Geometry check sheet. Reference: the model listing, model coordinates, mm. Round coordinates to 2 decimals unless told otherwise and drop trailing zeros. Order: outer loops, then holes, each group sorted by start corner. A loop starts at its lowest first (then second) coordinate and runs counter-clockwise, first axis right, second up. Notation, with made-up numbers: (17.25, -39.75) - (58.25, -39.75) arc R22 ccw to (58.25, -3.75) - close; hole circle Ø6 at (21, 15.25). An arc over 180 degrees is marked (long way). Write each question's results on one line, items separated by ' | '.
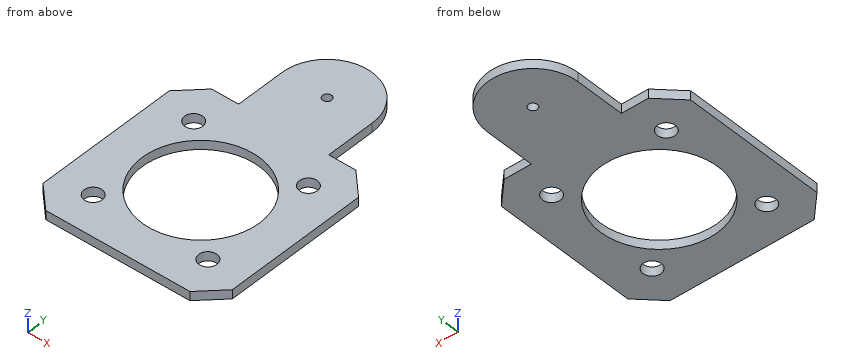
```python
from build123d import *

# Parameters (mm, degrees)
CROQUIS1_R              = 2
CROQUIS1_R_2            = 13
CROQUIS1_R_3            = 1
SALIENTE_EXTRUIR1_DEPTH = 2


with BuildPart() as part:
    # Croquis1 → Saliente-Extruir1 (new body)
    with BuildSketch(Plane.XY):
        with BuildLine():
            Line((10, 21), (16, 21))
            Line((16, 21), (21, 16))
            Line((21, 16), (21, -16))
            Line((21, -16), (16, -21))
            Line((16, -21), (-16, -21))
            Line((-16, -21), (-21, -16))
            Line((-21, -16), (-21, 16))
            Line((-21, 16), (-16, 21))
            Line((-16, 21), (-10, 21))
            Line((-10, 21), (-10, 32))
            ThreePointArc((-10, 32), (0, 42), (10, 32))
            Line((10, 32), (10, 21))
        make_face()
        with Locations((12.727922061, 12.727922061)):
            Circle(CROQUIS1_R, mode=Mode.SUBTRACT)
        with Locations((12.727922061, -12.727922061)):
            Circle(CROQUIS1_R, mode=Mode.SUBTRACT)
        with Locations((-12.727922061, -12.727922061)):
            Circle(CROQUIS1_R, mode=Mode.SUBTRACT)
        with Locations((-12.727922061, 12.727922061)):
            Circle(CROQUIS1_R, mode=Mode.SUBTRACT)
        Circle(CROQUIS1_R_2, mode=Mode.SUBTRACT)
        with Locations((0, 32)):
            Circle(CROQUIS1_R_3, mode=Mode.SUBTRACT)
    extrude(amount=SALIENTE_EXTRUIR1_DEPTH)


solid = part.part
```
(1) Depth check by flat-ended pin: pin 1 Ø2.5 at (x, y) = (12.73, 12.73) entering from +Z. Enter the tip coordinate at first touch or a pass-through.
Answers follow:
pin 1: through
(2) Material ranges on line 1 (Y direction, x = 0, z = 0.4); line 2 (X direction, y = -11.5, z = 1.95); line 3 (Y direction, x = -14, z = 0.3), recorded low to high.
Answers follow:
line 1: -21 to -13, 13 to 31, 33 to 42 | line 2: -21 to -14.31, -11.15 to -6.06, 6.06 to 11.15, 14.31 to 21 | line 3: -21 to -14.27, -11.18 to 11.18, 14.27 to 21
(3) Section check D-D (y = -9.5). Record the cut outline in (x, z).
Answers follow:
outline: (-21, 0) - (-8.87, 0) - (-8.87, 2) - (-21, 2) - close; (8.87, 0) - (21, 0) - (21, 2) - (8.87, 2) - close
(4) Section check A-A (x = 0). Record the cut outline in (y, z), then the cut area to 3 significant figures.
Answers follow:
outline: (-21, 0) - (-13, 0) - (-13, 2) - (-21, 2) - close; (13, 0) - (31, 0) - (31, 2) - (13, 2) - close; (33, 0) - (42, 0) - (42, 2) - (33, 2) - close | area: 70.0 mm²
(5) Section check C-C (z = 0.3). Record the cut outline in (x, y), then the cut area to 3 significant figures.
Answers follow:
outline: (-21, -16) - (-16, -21) - (16, -21) - (21, -16) - (21, 16) - (16, 21) - (10, 21) - (10, 32) arc R10 ccw to (-10, 32) - (-10, 21) - (-16, 21) - (-21, 16) - close; hole circle Ø4 at (-12.73, -12.73); hole circle Ø4 at (-12.73, 12.73); hole circle Ø26 at (0, 0); hole circle Ø2 at (0, 32); hole circle Ø4 at (12.73, -12.73); hole circle Ø4 at (12.73, 12.73) | area: 1,510 mm²
(6) Section check B-B (y = 0). Record the cut outline in (x, z), then the cut area to 3 significant figures.
Answers follow:
outline: (-21, 0) - (-13, 0) - (-13, 2) - (-21, 2) - close; (13, 0) - (21, 0) - (21, 2) - (13, 2) - close | area: 32.0 mm²
